Model file for the job. Use its own axes, mm. Face numbers are marked on the shaded views. A direction names the side the tool comes from. Give positions to 0.01 mm unless a question says otherwise; leave off trailing zeros. Write each loop counter-clockwise with the first axis right and the second up, starting at its lowest first coordinate (ties: lowest second). Pieces come first, ordered by that corner, then holes. Notation, with made-up numbers: (87, -15.75) - (102, -15.75) arc R31 cw to (102, 18.25) - close; hole circle Ø6 at (-20.75, 20.5). An arc over 180 degrees is marked (long way). Use CSV: the item, a comma, the result in double quotes.
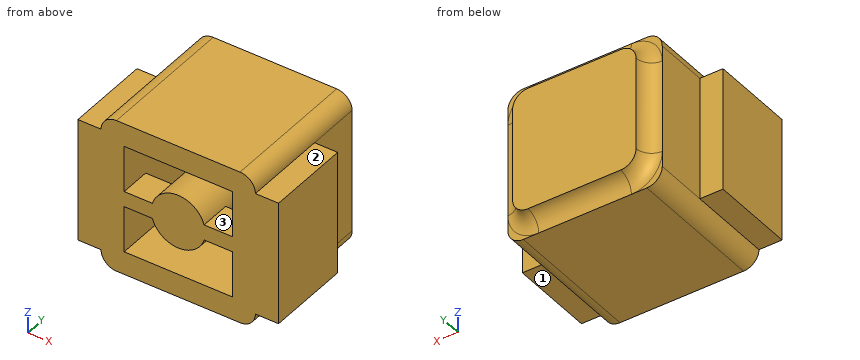
from build123d import *

# Parameters (mm, degrees)
BOSS_EXTRUDE1_DEPTH = 10
SKETCH2_W           = 13
SKETCH2_H           = 8
BOSS_EXTRUDE2_DEPTH = 5.5
SKETCH3_W           = 7
SKETCH3_H           = 7
SKETCH3_R           = 1.75
CUT_EXTRUDE1_DEPTH  = 8
SKETCH4_W           = 1
SKETCH4_H           = 2
BOSS_EXTRUDE3_DEPTH = 7
SKETCH5_W           = 10
SKETCH5_H           = 10
SKETCH5_W_2         = 8
SKETCH5_H_2         = 8
CUT_EXTRUDE2_DEPTH  = 1
FILLET1_R           = 1


with BuildPart() as part:
    # Sketch1 → Boss-Extrude1 (new body)
    with BuildSketch(Plane(origin=(0, 0, 0), x_dir=(1, 0, 0), z_dir=(0, 1, 0))):
        with BuildLine():
            Line((-4, -5), (4, -5))
            ThreePointArc((4, -5), (4.707106781, -4.707106781), (5, -4))
            Line((5, -4), (5, 4))
            ThreePointArc((5, 4), (4.707106781, 4.707106781), (4, 5))
            Line((4, 5), (-4, 5))
            ThreePointArc((-4, 5), (-4.707106781, 4.707106781), (-5, 4))
            Line((-5, 4), (-5, -4))
            ThreePointArc((-5, -4), (-4.707106781, -4.707106781), (-4, -5))
        make_face()
    extrude(amount=BOSS_EXTRUDE1_DEPTH)

    # Sketch2 → Boss-Extrude2 (add)
    with BuildSketch(Plane(origin=(0, 0, 0), x_dir=(1, 0, 0), z_dir=(0, 1, 0))):
        Rectangle(SKETCH2_W, SKETCH2_H)
    extrude(amount=BOSS_EXTRUDE2_DEPTH)

    # Sketch3 → Cut-Extrude1 (cut)
    with BuildSketch(Plane.XZ):
        Rectangle(SKETCH3_W, SKETCH3_H)
        with Locations(Location((0, 0, 0), (0, 0, 270))):
            Circle(SKETCH3_R, mode=Mode.SUBTRACT)
    extrude(amount=-CUT_EXTRUDE1_DEPTH, mode=Mode.SUBTRACT)

    # Sketch4 → Boss-Extrude3 (add)
    with BuildSketch(Plane(origin=(-3.5, 0, 0), x_dir=(0, 0, -1), z_dir=(1, 0, 0))):
        with Locations((0, 1)):
            Rectangle(SKETCH4_W, SKETCH4_H)
    extrude(amount=BOSS_EXTRUDE3_DEPTH)

    # Sketch5 → Cut-Extrude2 (cut)
    with BuildSketch(Plane(origin=(0, 10, 0), x_dir=(1, 0, 0), z_dir=(0, 1, 0))):
        Rectangle(SKETCH5_W, SKETCH5_H)
        Rectangle(SKETCH5_W_2, SKETCH5_H_2, mode=Mode.SUBTRACT)
    extrude(amount=-CUT_EXTRUDE2_DEPTH, mode=Mode.SUBTRACT)

    # Fillet1
    fillet1_edges = [part.edges().sort_by_distance(p)[0] for p in [
        (-4, 9, 0),
        (0, 9, 4),
        (4, 9, 0),
        (0, 9, -4),
        (-4, 9.5, -4),
        (4, 9.5, -4),
        (4, 9.5, 4),
        (-4, 9.5, 4),
    ]]
    fillet(fillet1_edges, radius=FILLET1_R - 0.0001)  # a hair under: the kernel refuses the full size


solid = part.part
(1) Saw through at B-B, the plane y = 7.5. List the corners of the cut face in (x, z).
Checked values:
outline,"(-5, -4) arc R1 ccw to (-4, -5) - (4, -5) arc R1 ccw to (5, -4) - (5, 4) arc R1 ccw to (4, 5) - (-4, 5) arc R1 ccw to (-5, 4) - close; circle Ø3.5 at (0, 0); hole (-3.5, -3.5) - (3.5, -3.5) - (3.5, 3.5) - (-3.5, 3.5) - close"
(2) Saw through at D-D, the plane y = 8.5. List the corners of the cut face in (x, z), then the cut area to 3 significant figures.
Checked values:
outline,"(-5, -4) arc R1 ccw to (-4, -5) - (4, -5) arc R1 ccw to (5, -4) - (5, 4) arc R1 ccw to (4, 5) - (-4, 5) arc R1 ccw to (-5, 4) - close"
area,"99.1 mm^2"
(3) Wall check: probe 1 along Z at (x, y) = (-3.25, 1.25); probe 2 along X at (y, z) = (4, -2.25); probe 3 along X at (y, z) = (2.75, 0.5). Give the ranges that are in metal, low to high. Write a range as [from, to].
Checked values:
probe 1,"z = [-5, -3.5], [-0.5, 0.5], [3.5, 5]"
probe 2,"x = [-6.5, -3.5], [3.5, 6.5]"
probe 3,"x = [-6.5, -3.5], [-1.68, 1.68], [3.5, 6.5]"
(4) 3-axis set-ups, long thin cutter, end or side, ignore diameter. For the marked faces 1, 2 and 3: which of +Z, -Z, +X, -X, +Y, -Y reach the whole face in a straight line?
Checked values:
face 1,"-Z, +X, +Y, -Y"
face 2,"+Z, +X, +Y, -Y"
face 3,"-Y"
(5) Flat gauge pins, fed straight in: P1, Ø2, axis at y = 6, z = 1.5, coming from the -X side; P2, Ø1.2, axis at x = -6, z = 1.5, coming from the +Y side; P3, Ø1.2, axis at x = 6, y = 1.5, coming from the +Z side. Where does each tip first touch, or does it go through?
Checked values:
P1,"stops at x = -6.5"
P2,"stops at y = 5.5"
P3,"stops at z = 4"
